Source: CAD feature listing. Evaluate the final solid. Frame: model axes, mm. A direction names the side the tool comes from. Round coordinates to 2 decimals unless told otherwise and drop trailing zeros. Loops run counter-clockwise (first coordinate to the right, second up) from the corner with the lowest first, then second, coordinate; pieces in that order, holes last. Notation, with made-up numbers: (73, -21.75) - (106, -21.75) arc R17 ccw to (106, -16.75) - close; hole circle Ø10 at (63.25, -30.5). An arc over 180 degrees is marked (long way). One line per question, with ' | ' between items. Start each with the question number.
1. Cut plane B-B (y = 0). Return loops of the section in (x, z), then the cut area to 3 significant figures.
2. Pin query (flat end, axial travel): pin 1 (17.5 mm diameter, centred on x = -20, z = -2.5, fed in from -Y); pin 2 (0.6 mm diameter, centred on x = -30.5, z = 12, fed in from +Y); pin 3 (2 mm diameter, centred on x = -30, y = -0.5, fed in from +Z). Return the tip coordinate at first contact, or that it passes through.
3. Mould query, pull axis Y, two halves, no side actions, for faces 1 (the flat face through (-6.389, 5, 0)), 2 (the flat face through (-30, 0, 7.936)), 3 (the flat face through (-3, 11.43, 0)). Classes: pulls with the +Y half, pulls with the -Y half, needs draft (parallel to the pull), parting line crosses it, or undercut.
4. Cut plane A-A (y = 10.5). Return loops of the section in (x, z), then the cut area to 3 significant figures.
5. Cut plane C-C (z = 17). Return loops of the section in (x, y), then the cut area to 3 significant figures.
6. Ray query, line 1 (Z direction, x = -21, y = -1.5); line 2 (Y direction, x = -8.5, z = -7); line 3 (X direction, y = 4.5, z = 8). Return the intervals inside material, ascending.
7. Cut plane D-D (z = -8). Return loops of the section in (x, y), then the cut area to 3 significant figures.
8. Access query for faces 4 (the flat face through (-18, 3, -1)), 5 (the flat face through (-18, -3, -1)), 6 (the flat face through (-30, -3.974, 11)), 7 (the flat face through (-5.3, 0.1, 10.16)). Directions: +Z, -Z, +X, -X, +Y, -Y. A direction counts if a zero-diameter tool reaches every point of the face in a straight line with its end or side. Return the directions, or none.
```python
from build123d import *

# Parameters (mm, degrees)
BOSS_EXTRUDE1_DEPTH = 19.05
SKETCH6_W           = 16.071399664
SKETCH6_H           = 6
BOSS_EXTRUDE3_DEPTH = 23
SKETCH3_W           = 2.54
SKETCH3_H           = 5.08
SKETCH4_R           = 15.5
SKETCH4_R_2         = 1.099962386
SKETCH4_R_3         = 1.0993224
SKETCH4_W           = 8
SKETCH4_H           = 6
BOSS_EXTRUDE2_DEPTH = 2
FILLET1_R           = 1


with BuildPart() as part:
    # Sketch1 → Boss-Extrude1 (new body, symmetric)
    with BuildSketch(Plane.XY):
        with BuildLine():
            Line((8.346153406, -9.946558305), (7.464020663, -14.949381691))
            ThreePointArc((7.464020663, -14.949381691), (3.546652059, -13.692553844), (0.110630651, -11.43))
            Line((0.110630651, -11.43), (-6.389369349, -11.43))
            Line((-6.389369349, -11.43), (-6.389369349, 11.43))
            Line((-6.389369349, 11.43), (0.110630651, 11.43))
            ThreePointArc((0.110630651, 11.43), (3.546652059, 13.692553844), (7.464020663, 14.949381691))
            Line((7.464020663, 14.949381691), (8.346153406, 9.946558305))
            ThreePointArc((8.346153406, 9.946558305), (0, 0), (8.346153406, -9.946558305))
        make_face()
    extrude(amount=BOSS_EXTRUDE1_DEPTH, both=True)

    # Sketch6 → Boss-Extrude3 (add)
    with BuildSketch(Plane.ZY.offset(6.389369349)):
        with Locations((-1.213689559, 0)):
            Rectangle(SKETCH6_W, SKETCH6_H)
    extrude(amount=BOSS_EXTRUDE3_DEPTH)

    # Sketch3 → Cut-Revolve1 (revolve, cut)
    with BuildSketch(Plane(origin=(0, 0, 0), x_dir=(1, 0, 0), z_dir=(0, 1, 0))):
        with Locations((-6.35, 12.7)):
            Rectangle(SKETCH3_W, SKETCH3_H)
        with Locations((-6.35, -12.7)):
            Rectangle(SKETCH3_W, SKETCH3_H)
    revolve(axis=Axis((10.1, 0, 19.05), (0, 0, -1)), mode=Mode.SUBTRACT)

    # Sketch4 → Boss-Extrude2 (add)
    with BuildSketch(Plane(origin=(-29.389369349, 0, 0), x_dir=(0, -1, 0), z_dir=(-1, 0, 0))):
        Circle(SKETCH4_R)
        with Locations((6.97426488, 10.435972737)):
            Circle(SKETCH4_R_2, mode=Mode.SUBTRACT)
        with Locations((-8.02573512, -8.580948715)):
            Circle(SKETCH4_R_3, mode=Mode.SUBTRACT)
        with Locations((-0.025715642, 10.93618237)):
            Rectangle(SKETCH4_W, SKETCH4_H, mode=Mode.SUBTRACT)
    extrude(amount=BOSS_EXTRUDE2_DEPTH)

    # Fillet1
    fillet1_edges = [part.edges().sort_by_distance(p)[0] for p in [
        (-6.389369349, 0, 19.05),
        (-6.389369349, 0, -19.05),
    ]]
    fillet(fillet1_edges, radius=FILLET1_R)


solid = part.part
```
Answers follow:
1) outline: (-31.39, -15.5) - (-29.39, -15.5) - (-29.39, -9.25) - (-6.39, -9.25) - (-6.39, -10.16) - (-5.08, -10.16) - (-5.08, -15.24) - (-6.39, -15.24) - (-6.39, -18.05) arc R1 ccw to (-5.39, -19.05) - (0, -19.05) - (0, 19.05) - (-5.39, 19.05) arc R1 ccw to (-6.39, 18.05) - (-6.39, 15.24) - (-5.08, 15.24) - (-5.08, 10.16) - (-6.39, 10.16) - (-6.39, 6.82) - (-29.39, 6.82) - (-29.39, 7.94) - (-31.39, 7.94) - close; (-31.39, 13.94) - (-29.39, 13.94) - (-29.39, 15.5) - (-31.39, 15.5) - close | area: 649 mm2
2) pin 1: stops at y = -3 | pin 2: stops at y = 10.17 | pin 3: stops at z = 15.5
3) face 1: needs draft | face 2: undercut | face 3: pulls with the +Y half
4) outline: (-31.39, -11.4) - (-29.39, -11.4) - (-29.39, 11.4) - (-31.39, 11.4) - close; (-6.39, -18.05) arc R1 ccw to (-5.39, -19.05) - (8.25, -19.05) - (8.25, 19.05) - (-5.39, 19.05) arc R1 ccw to (-6.39, 18.05) - close; hole (-4.17, -15.24) - (-0.86, -15.24) - (-0.86, -10.16) - (-4.17, -10.16) - close; hole (-4.17, 10.16) - (-0.86, 10.16) - (-0.86, 15.24) - (-4.17, 15.24) - close | area: 569 mm2
5) outline: (-6.39, -11.43) - (0.11, -11.43) arc R15.18 ccw to (7.46, -14.95) - (8.35, -9.95) arc R10.1 cw to (8.35, 9.95) - (7.46, 14.95) arc R15.18 ccw to (0.11, 11.43) - (-6.39, 11.43) - close | area: 246 mm2
6) line 1: z = -9.25 to 6.82 | line 2: y = -3 to 3 | line 3: x = -31.39 to -29.39, -6.39 to 1.06
7) outline: (-31.39, -13.28) - (-29.39, -13.28) - (-29.39, -3) - (-6.39, -3) - (-6.39, -11.43) - (0.11, -11.43) arc R15.18 ccw to (7.46, -14.95) - (8.35, -9.95) arc R10.1 cw to (8.35, 9.95) - (7.46, 14.95) arc R15.18 ccw to (0.11, 11.43) - (-6.39, 11.43) - (-6.39, 3) - (-29.39, 3) - (-29.39, 7.09) - (-31.39, 7.09) - close; (-31.39, 8.96) - (-29.39, 8.96) - (-29.39, 13.28) - (-31.39, 13.28) - close | area: 433 mm2
8) face 4: +Z, -Z, +Y | face 5: +Z, -Z, -Y | face 6: -X | face 7: none
